The model under review builds one solid part; all positions refer to its coordinate system, in mm. Face numbers are marked on the shaded views. Coordinates: 2 decimals unless noted, no trailing zeros. Order: outer loops, then holes, each group sorted by start corner. A loop starts at its lowest first (then second) coordinate and runs counter-clockwise, first axis right, second up. Notation, with made-up numbers: (48, 35.25) -> (62, 35.25) arc R13 ccw to (62, 59.25) -> close; hole circle Ø10 at (-38, 64.5). An arc over 180 degrees is marked (long way). Use CSV: the item, a comma, the result in double quotes. Start each with the question number.
```python
from build123d import *

# Parameters (mm, degrees)
F0_R          = 60
F0_R_2        = 59
F1_DEPTH      = 80
F1_DEPTH_BACK = 80
F2_R          = 1.5
F3_DEPTH      = 59.0000001
F3_DEPTH_BACK = 59.0000001
F4_R          = 5
F5_DEPTH      = 2.2456623517
F5_DEPTH_BACK = 7.6787548984
F6_DEPTH      = 60.001


with BuildPart() as f1:
    # F0 (on Front) → F1 (new body, two sides)
    with BuildSketch(Plane.XZ) as f1_sk:
        Circle(F0_R)
        Circle(F0_R_2, mode=Mode.SUBTRACT)
    extrude(amount=F1_DEPTH)
    extrude(f1_sk.sketch, amount=-F1_DEPTH_BACK)

    # F2 (on Top) → F3 (join, two sides)
    with BuildSketch(Plane.XY) as f3_sk:
        with BuildLine():
            add(Edge.make_bspline(
                [(0, -50), (-3.3022109419, -31.783785671), (-2.6830465067, 18.5749381781), (0, 50)],
                knots=[0, 0, 0, 0, 100, 100, 100, 100], degree=3))
            add(Edge.make_bspline(
                [(0, -50), (16.5110565722, -50.1523353159), (7.2235865518, 0), (0, 50)],
                knots=[0, 0, 0, 0, 100, 100, 100, 100], degree=3))
        make_face()
        with Locations((2.4201369379, 0)):
            Circle(F2_R, mode=Mode.SUBTRACT)
        with Locations((2.4201369379, 0)):
            Circle(F2_R)
    extrude(amount=F3_DEPTH)
    extrude(f3_sk.sketch, amount=-F3_DEPTH_BACK)

    # F4 (on Right) → F5 (cut, two sides)
    with BuildSketch(Plane.YZ) as f5_sk:
        Circle(F4_R)
    extrude(amount=-F5_DEPTH, mode=Mode.SUBTRACT)
    extrude(f5_sk.sketch, amount=F5_DEPTH_BACK, mode=Mode.SUBTRACT)

    # F2 (on Top) → F6 (cut, through all)
    with BuildSketch(Plane.XY):
        with Locations((2.4201369379, 0)):
            Circle(F2_R)
    extrude(amount=F6_DEPTH, mode=Mode.SUBTRACT)


solid = f1.part
```
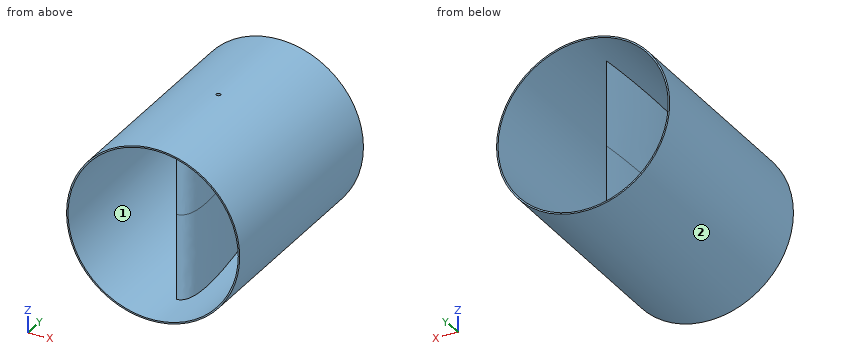
Q1. Add section A-A, the plane x = 25.5. State the section outline as (y, z) points, then the cut area to 3 significant figures.
Q2. Clearance check with flat-ended pins moving along their axes: pin 1 Ø1.5 at (x, y) = (24, 0) entering from -Z; pin 2 Ø10 at (x, y) = (9, 8.5) entering from -Z; pin 3 Ø2 at (y, z) = (-38.5, 9) entering from -X; pin 4 Ø12 at (x, z) = (47, -4.5) entering from -Y. State where each tip first meets the part, or that it passes through.
Q3. Add section B-B, the plane z = 7. State how many separate pieces and enclosed holes the cut face has, then the cut area to 3 significant figures.
Q4. Add section C-C, the plane y = 63.5. State the section outline as (x, z) points.
Q5. Draft analysis for pull direction Z (two halves, no side actions). For the marked faces 1 and 2, state which applies: +Z half, -Z half, draft (parallel to the pull), parting line (faces both ways), or undercut.
Q6. To check wall thickness, follow probe 1 along X at (y, z) = (30, 27); probe 2 along X at (y, z) = (11, -53.5); probe 3 along X at (y, z) = (0, 44). State the ranges of each line that lie inside material, in increasing order.
Answer block:
1,outline,"(-80, -54.31) -> (80, -54.31) -> (80, -53.2) -> (-80, -53.2) -> close; (-80, 53.2) -> (80, 53.2) -> (80, 54.31) -> (-80, 54.31) -> close"
1,area,"354 mm²"
2,pin 1,"stops at z = -55.31"
2,pin 2,"stops at z = -59.87"
2,pin 3,"stops at x = -59.46"
2,pin 4,"passes through"
3,separate pieces,"3"
3,enclosed holes,"1"
3,area,"1,060 mm²"
4,outline,"circle Ø120 at (0, 0); hole circle Ø118 at (0, 0)"
5,face 1,"undercut"
5,face 2,"parting line"
6,probe 1,"x = -53.58 to -52.46, -1.31 to 2.95, 52.46 to 53.58"
6,probe 2,"x = -27.16 to -24.87, -2.01 to 5.68, 24.87 to 27.16"
6,probe 3,"x = -40.79 to -39.31, -2.21 to 0.92, 3.92 to 7.1, 39.31 to 40.79"
